```python
from build123d import *

# Parameters (mm, degrees)
F1_DEPTH       = 31.75
F2_R           = 14.325
F3_DEPTH       = 28.575
F5_DEPTH       = 31.75
F7_DEPTH       = 31.751
F9_DEPTH       = 31.751
F10_W          = 27.8922222136
F10_H          = 28.1136979927
F10_W_2        = 22.0070765571
F10_H_2        = 22.18663187
F10_W_3        = 19.4776418147
F10_H_3        = 19.6770581923
F10_W_4        = 24.7722447466
F10_H_4        = 25.0182185186
F11_DEPTH      = 31.75
F12_R          = 1.524
F13_R          = 1.524
F14_R          = 3.175
F16_DEPTH      = 31.75
F20_DEPTH      = 131.1291589461
F20_DEPTH_BACK = 124.3230200021
F21_R          = 3.5
F21_R_2        = 1.75
F22_DEPTH      = 31.751


# Not quite as in the source:
# - a feature names something its author has since deleted; it is built from what else it names


with BuildPart() as f1:
    # F0 (on Top) → F1 (new body)
    with BuildSketch(Plane.XY):
        with BuildLine():
            ThreePointArc((-171.2164076011, 147.819121873), (-151.8134645157, 142.5585953186), (-140.2663976585, 159.0149797027))
            ThreePointArc((-140.2663976585, 159.0149797027), (-141.8914670948, 166.3795285416), (-146.4648638984, 172.3763170112))
            ThreePointArc((-146.4648638984, 172.3763170112), (-170.0918974756, 171.438024992), (-171.2164076011, 147.819121873))
        make_face()
        with BuildLine():
            ThreePointArc((-146.4648638984, 172.3763170112), (-141.8914670948, 166.3795285416), (-140.2663976585, 159.0149797027))
            ThreePointArc((-140.2663976585, 159.0149797027), (-151.8134645157, 142.5585953186), (-171.2164076011, 147.819121873))
            Line((-171.2164076011, 147.819121873), (-48.1710061431, 0))
            Line((-48.1710061431, 0), (0, 0))
            Line((0, 0), (0, 48.4906934548))
            Line((0, 48.4906934548), (-146.4648638984, 172.3763170112))
        make_face()
    extrude(amount=F1_DEPTH)

    # F2 (on face) → F3 (cut)
    with BuildSketch(Plane.XY.offset(31.75)):
        with Locations((-157.7663976585, 159.0149797027)):
            Circle(F2_R)
    extrude(amount=-F3_DEPTH, mode=Mode.SUBTRACT)

    # F4 (on face) → F5 (join)
    with BuildSketch(Plane.XY.offset(31.75)):
        Polygon((-11.849261314, 0), (-36.3217448291, 0), (-41.8210061431, -9.525), (-6.35, -9.525), align=None)
    extrude(amount=-F5_DEPTH)

    # F6 (on face) → F7 (cut, through all)
    with BuildSketch(Plane.XY.offset(31.75)):
        Polygon((-9.652, 6.223), (0, 11.7955847982), (0, 36.6951086566), (-9.652, 42.2676934548), align=None)
    extrude(amount=-F7_DEPTH, mode=Mode.SUBTRACT)

    # F8 (on face) → F9 (cut, through all)
    with BuildSketch(Plane.XY.offset(31.75)):
        with BuildLine():
            Line((-16.002, 49.699371019), (-140.6956326235, 162.8671195132))
            ThreePointArc((-140.6956326235, 162.8671195132), (-140.3740374375, 160.9529698843), (-140.2663976585, 159.0149797027))
            ThreePointArc((-140.2663976585, 159.0149797027), (-146.8924666341, 145.3033924833), (-161.7529832673, 141.9751107131))
            Line((-161.7529832673, 141.9751107131), (-40.600106963, 6.35))
            Line((-40.600106963, 6.35), (-16.002, 6.35))
            Line((-16.002, 6.35), (-16.002, 49.699371019))
        make_face()
    extrude(amount=-F9_DEPTH, mode=Mode.SUBTRACT)

    # F10 (on face) → F11 (join, through all)
    with BuildSketch(Plane.XY.offset(31.75)):
        with BuildLine():
            ThreePointArc((-144.01445162, 148.1921344135), (-145.4358718483, 146.5969229609), (-147.0410978414, 145.1868220585))
            Line((-147.0410978414, 145.1868220585), (-147.0410978414, 125.5058270234))
            Line((-147.0410978414, 125.5058270234), (-144.0114513942, 122.1142762212))
            Line((-144.0114513942, 122.1142762212), (-124.3630560267, 122.1142762212))
            Line((-124.3630560267, 122.1142762212), (-124.3630560267, 100.1187951534))
            Line((-124.3630560267, 100.1187951534), (-121.3334095795, 96.7272443512))
            Line((-121.3334095795, 96.7272443512), (-99.1555794696, 96.7272443512))
            Line((-99.1555794696, 96.7272443512), (-99.1555794696, 71.9001766348))
            Line((-99.1555794696, 71.9001766348), (-96.1259330223, 68.5086258326))
            Line((-96.1259330223, 68.5086258326), (-71.182934723, 68.5086258326))
            Line((-71.182934723, 68.5086258326), (-71.182934723, 40.5860786421))
            Line((-71.182934723, 40.5860786421), (-68.1532882758, 37.1945278399))
            Line((-68.1532882758, 37.1945278399), (-40.0903125094, 37.1945278399))
            Line((-40.0903125094, 37.1945278399), (-40.0903125094, 6.35))
            Line((-40.0903125094, 6.35), (-36.8899125094, 6.35))
            Line((-36.8899125094, 6.35), (-36.8899125094, 37.1945278399))
            Line((-36.8899125094, 37.1945278399), (-16.002, 37.1945278399))
            Line((-16.002, 37.1945278399), (-16.002, 40.3949278399))
            Line((-16.002, 40.3949278399), (-36.8899125094, 40.3949278399))
            Line((-36.8899125094, 40.3949278399), (-36.8899125094, 68.6565381148))
            Line((-36.8899125094, 68.6565381148), (-40.2532893295, 71.7090258326))
            Line((-40.2532893295, 71.7090258326), (-67.982534723, 71.7090258326))
            Line((-67.982534723, 71.7090258326), (-67.982534723, 96.8751566334))
            Line((-67.982534723, 96.8751566334), (-71.3459115431, 99.9276443512))
            Line((-71.3459115431, 99.9276443512), (-95.9551794696, 99.9276443512))
            Line((-95.9551794696, 99.9276443512), (-95.9551794696, 122.2621885034))
            Line((-95.9551794696, 122.2621885034), (-99.3185562896, 125.3146762212))
            Line((-99.3185562896, 125.3146762212), (-121.1626560267, 125.3146762212))
            Line((-121.1626560267, 125.3146762212), (-121.1626560267, 145.1396466957))
            Line((-121.1626560267, 145.1396466957), (-124.5260328468, 148.1921344135))
            Line((-124.5260328468, 148.1921344135), (-144.01445162, 148.1921344135))
        make_face()
        with Locations((-54.0364236162, 54.4517768362)):
            Rectangle(F10_W, F10_H, mode=Mode.SUBTRACT)
        with Locations((-110.1591177481, 111.0209602862)):
            Rectangle(F10_W_2, F10_H_2, mode=Mode.SUBTRACT)
        with Locations((-134.101876934, 135.1532053173)):
            Rectangle(F10_W_3, F10_H_3, mode=Mode.SUBTRACT)
        with Locations((-83.5690570963, 84.2181350919)):
            Rectangle(F10_W_4, F10_H_4, mode=Mode.SUBTRACT)
    extrude(amount=-F11_DEPTH)

    # F12
    f12_edges = [f1.edges().sort_by_distance(p)[0] for p in [
        (-147.041098, 145.186822, 15.875),
        (-161.752983, 141.975111, 15.875),
        (-147.041098, 125.505827, 15.875),
        (-140.695633, 162.86712, 15.875),
        (-144.014452, 148.192134, 15.875),
        (-124.526033, 148.192134, 15.875),
    ]]
    fillet(f12_edges, radius=F12_R)

    # F13
    f13_edges = [f1.edges().sort_by_distance(p)[0] for p in [
        (-124.363056, 100.118795, 15.875),
        (-144.011451, 122.114276, 15.875),
        (-121.33341, 96.727244, 15.875),
        (-99.155579, 71.900177, 15.875),
        (-71.182935, 40.586079, 15.875),
        (-96.125933, 68.508626, 15.875),
        (-95.955179, 122.262189, 15.875),
        (-121.162656, 145.139647, 15.875),
        (-67.982535, 96.875157, 15.875),
        (-99.318556, 125.314676, 15.875),
        (-71.345912, 99.927644, 15.875),
        (-40.253289, 71.709026, 15.875),
        (-68.153288, 37.194528, 15.875),
        (-36.889913, 68.656538, 15.875),
    ]]
    fillet(f13_edges, radius=F13_R)

    # F14
    f14_edges = [f1.edges().sort_by_distance(p)[0] for p in [
        (-40.090313, 40.394928, 15.875),
        (-67.982535, 40.394928, 15.875),
        (-67.982535, 68.508626, 15.875),
        (-40.090313, 68.508626, 15.875),
        (-40.090313, 37.194528, 15.875),
        (-16.002, 37.194528, 15.875),
        (-36.889913, 37.194528, 15.875),
        (-36.889913, 6.35, 15.875),
        (-16.002, 6.35, 15.875),
        (-71.182935, 68.508626, 15.875),
        (-71.182935, 71.709026, 15.875),
        (-67.982535, 71.709026, 15.875),
        (-95.955179, 71.709026, 15.875),
        (-95.955179, 96.727244, 15.875),
        (-71.182935, 96.727244, 15.875),
        (-99.155579, 96.727244, 15.875),
        (-99.155579, 122.114276, 15.875),
        (-124.363056, 122.114276, 15.875),
        (-124.363056, 144.991734, 15.875),
        (-95.955179, 99.927644, 15.875),
        (-121.162656, 99.927644, 15.875),
        (-143.840698, 125.314676, 15.875),
        (-99.155579, 99.927644, 15.875),
        (-124.363056, 125.314676, 15.875),
        (-121.162656, 122.114276, 15.875),
        (-143.840698, 144.991734, 15.875),
        (-36.889913, 40.394928, 15.875),
        (-16.002, 49.699371, 15.875),
        (-16.002, 40.394928, 15.875),
    ]]
    fillet(f14_edges, radius=F14_R)

    # F15 (on face) → F16 (join, through all)
    with BuildSketch(Plane.XY.offset(31.75)):
        with BuildLine():
            ThreePointArc((-40.0903125094, 9.9726537321), (-41.119997319, 8.4776111048), (-42.8839038824, 8.9066063266))
            Line((-42.8839038824, 8.9066063266), (-40.600106963, 6.35))
            Line((-40.600106963, 6.35), (-40.0903125094, 6.35))
            Line((-40.0903125094, 6.35), (-40.0903125094, 9.9726537321))
        make_face()
    extrude(amount=-F16_DEPTH)

    # F19 (on face) → F20 (cut, two sides)
    with BuildSketch(Plane(origin=(0, 0, 0), x_dir=(-0.7043142753, 0.7098883022, 0), z_dir=(0.7098883022, 0.7043142753, 0))) as f20_sk:
        Polygon((241.5, 6.35), (241.5, 31.75), (225.5252254981, 31.75), (63.5, 31.75), align=None)
    extrude(amount=-F20_DEPTH, mode=Mode.SUBTRACT)
    extrude(f20_sk.sketch, amount=F20_DEPTH_BACK, mode=Mode.SUBTRACT)

    # F21 (on face) → F22 (cut, through all)
    with BuildSketch(Plane(origin=(0, 0, 0), x_dir=(1, 0, 0), z_dir=(0, 0, -1))):
        with Locations((-157.7663976585, -159.0149797027)):
            Circle(F21_R)
        with Locations((-152.1318834564, -153.3358732848)):
            Circle(F21_R_2)
        with Locations((-163.4009118606, -164.6940861207)):
            Circle(F21_R_2)
        with Locations((-151.0224587872, -165.7059653177)):
            Circle(F21_R_2)
        with Locations((-164.5103365298, -152.3239940878)):
            Circle(F21_R_2)
    extrude(amount=-F22_DEPTH, mode=Mode.SUBTRACT)


solid = f1.part
```
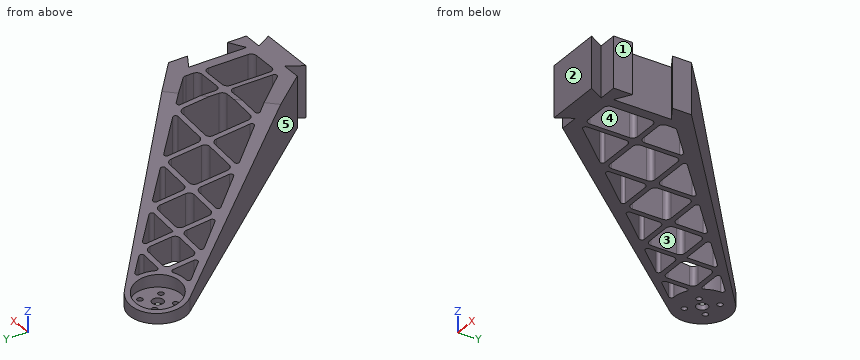
The model under review builds one solid part; all positions refer to its coordinate system, in mm. Face numbers are marked on the shaded views. A direction names the side the tool comes from. Give positions to 0.01 mm unless a question says otherwise; leave off trailing zeros. Write each loop counter-clockwise with the first axis right and the second up, starting at its lowest first coordinate (ties: lowest second). Pieces come first, ordered by that corner, then holes. Notation, with made-up numbers: (-8.5, 56) -> (-4.5, 56) arc R11 cw to (-4.5, 69) -> close; hole circle Ø9 at (31, 37). An arc over 180 degrees is marked (long way). Answer in a Markdown table with one row per item.
1) For L1, parallel to Y at x = -47.5, z = 24.5; L2, parallel to X at y = 49, z = 20; L3, parallel to Y at x = -21, z = 28 (3 decimals), list the stretches that pass through material, from the lowest coordinate up. Write a range as [from, to].
Worked answers:
| item | result |
|---|---|
| L1 | [0, 14.07], [37.19, 40.39], [68.51, 71.71], [78.29, 88.67] |
| L2 | [-88.96, -78.7], [-71.18, -67.98], [-40.09, -36.89], [-16.08, -0.6] |
| L3 | [-9.525, 6.35], [37.195, 40.395], [54.235, 66.253] |
2) Clearance check with flat-ended pins moving along their axes: P1, Ø12.5, axis at y = 113.5, z = 7, coming from the +X side; P2, Ø4, axis at y = 132.5, z = 4.5, coming from the -X side; P3, Ø14, axis at x = -131.5, z = 8, coming from the +Y side. State where each tip first meets the part, or that it passes through.
Worked answers:
| item | result |
|---|---|
| P1 | x = -69.47 |
| P2 | x = -160.13 |
| P3 | y = 165.64 |
3) Add section C-C on x = -25. State the section outline as (y, z) points (3 decimals), plus the area to 3 significant figures.
Worked answers:
| item | result |
|---|---|
| outline | (-9.525, 0) -> (6.35, 0) -> (6.35, 31.75) -> (-9.525, 31.75) -> close; (37.195, 0) -> (40.395, 0) -> (40.395, 31.75) -> (37.195, 31.75) -> close; (57.866, 0) -> (69.637, 0) -> (69.637, 31.245) -> (64.647, 31.75) -> (57.866, 31.75) -> close |
| area | 978 mm² |
4) Add section A-A on x = -88. State the section outline as (y, z) points.
Worked answers:
| item | result |
|---|---|
| outline | (47.85, 0) -> (59.41, 0) -> (59.41, 25.95) -> (47.85, 27.12) -> close; (68.51, 0) -> (71.71, 0) -> (71.71, 24.7) -> (68.51, 25.03) -> close; (96.73, 0) -> (99.93, 0) -> (99.93, 21.84) -> (96.73, 22.17) -> close; (115.04, 0) -> (122.92, 0) -> (122.92, 19.51) -> (115.04, 20.31) -> close |
5) Add section B-B on y = 83. State the section outline as (x, z) points.
Worked answers:
| item | result |
|---|---|
| outline | (-117.26, 0) -> (-109.07, 0) -> (-109.07, 21.44) -> (-117.26, 20.62) -> close; (-99.16, 0) -> (-95.96, 0) -> (-95.96, 22.76) -> (-99.16, 22.44) -> close; (-71.18, 0) -> (-67.98, 0) -> (-67.98, 25.57) -> (-71.18, 25.25) -> close; (-52.69, 0) -> (-40.8, 0) -> (-40.8, 28.3) -> (-52.69, 27.11) -> close |
6) Mouldability with a two-part tool opening along Y and no side actions: class the marked faces 1, 2 and 3 as +Y half, -Y half, draft (parallel to the pull), parting line (faces both ways), or undercut.
Worked answers:
| item | result |
|---|---|
| face 1 | draft |
| face 2 | -Y half |
| face 3 | undercut |
7) Tool access review of the marked faces 4 and 5: name each direction out of +Z, -Z, +X, -X, +Y, -Y from which nothing blocks a thin tool from reaching the whole face with its end or side.
Worked answers:
| item | result |
|---|---|
| face 4 | +Z, -Z |
| face 5 | +Z, -Z, -X, -Y |
